Part model, mm, in its own coordinate system. Face numbers are marked on the shaded views. A direction names the side the tool comes from. Coordinates: 2 decimals unless noted, no trailing zeros. Loops run counter-clockwise (first coordinate to the right, second up) from the corner with the lowest first, then second, coordinate; pieces in that order, holes last. Notation, with made-up numbers: (-32, -37.5) -> (-25, -37.5) arc R19 ccw to (-25, -7.5) -> close; hole circle Ø4 at (-35, 29). An arc over 180 degrees is marked (long way). One line per question, with ' | ' between items. Start each with the question number.
1) Drop flat-ended pins along their axis: pin 1 (3 mm diameter, centred on x = 3, z = -2, fed in from -Y); pin 2 (4 mm diameter, centred on x = -2, y = 2.5, fed in from -Z). Give the stop position or say it passes through.
2) 3-axis set-ups, long thin cutter, end or side, ignore diameter. For the marked faces 4 and 5: which of +Z, -Z, +X, -X, +Y, -Y reach the whole face in a straight line?
3) Cut at A-A (z = 4.25). List the corners of the cut face in (x, y).
4) Two-plate mould, pull along Z, no slides. Class the marked faces 1, 2 and 3: released by +Z, released by -Z, zero draft, split by the parting line, or undercut.
5) Probe L1, parallel to X at y = -1.5, z = 1.25; L2, parallel to X at y = 0.5, z = 4; L3, parallel to Z at x = 4.25, y = 0.5. List the from-to ranges inside material, lowest first. Write a range as from..to.
6) Cut at B-B (y = -3). List the corners of the cut face in (x, z), plus the area to 3 significant figures.
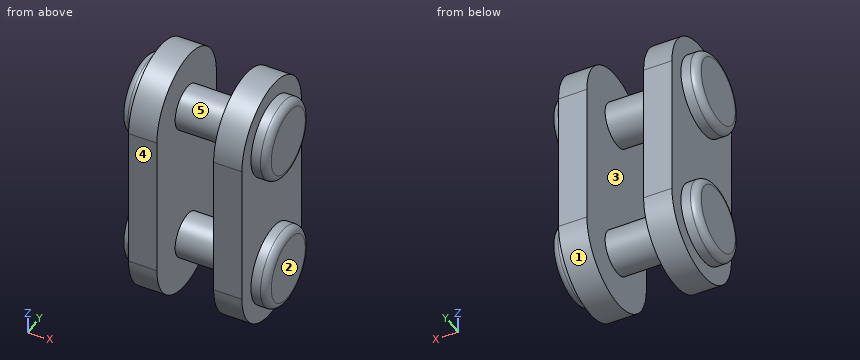
Autodesk Inventor part; units mm, degrees
ref_plane "ZS1_XY" through (0, 0, 0) normal (1, 0, 0) x (0, 0, -1)
ref_plane "ZS1_YZ" through (0, 0, 0) normal (0, 0, -1) x (0, 1, 0)
ref_plane "ZS1_ZX" through (0, 0, 0) normal (0, 1, 0) x (1, 0, 0)
sketch "Skizze_1" plane through (0, 0, 0) normal (0, 1, 0) x (-1, 0, 0)
  line L0 (4, 14.4) -> (2, 14.4)
  line L1 (2, 14.4) -> (2, -4)
  line L2 (2, -4) -> (4, -4)
  line L3 (4, -4) -> (4, 14.4)
extrude "Extrusion1" add sketch "Skizze_1" along normal mid plane 8
sketch "Skizze_2" plane through (0, 0, 0) normal (0, 1, 0) x (-1, 0, 0)
  line L0 (-5.17, 0) -> (0, 0)
  line L1 (5.17, 0) -> (5.17, -2.29)
  arc A0 (4.67, -2.79) -> (5.17, -2.29) centre (4.67, -2.29) ccw
  line L2 (4.67, -2.79) -> (4, -2.79)
  line L3 (4, -2.79) -> (4, -1.55)
  line L4 (4, -1.55) -> (-4, -1.55)
  line L5 (-4, -1.55) -> (-4, -2.79)
  line L6 (-4, -2.79) -> (-4.67, -2.79)
  arc A1 (-5.17, -2.29) -> (-4.67, -2.79) centre (-4.67, -2.29) ccw
  line L7 (-5.17, -2.29) -> (-5.17, 0)
  line L8 (-5.17, 0) -> (5.17, 0)
revolve "Revolution1" add sketch "Skizze_2" angle 360 about axis through (5.17, 0, 0) along (1, 0, 0)
sketch "Skizze_3" plane through (0, 0, 0) normal (0, 1, 0) x (-1, 0, 0)
  line L0 (-5.17, 10.4) -> (0, 10.4)
  line L1 (5.17, 10.4) -> (5.17, 8.11)
  arc A0 (4.67, 7.61) -> (5.17, 8.11) centre (4.67, 8.11) ccw
  line L2 (4.67, 7.61) -> (4, 7.61)
  line L3 (4, 7.61) -> (4, 8.85)
  line L4 (4, 8.85) -> (-4, 8.85)
  line L5 (-4, 8.85) -> (-4, 7.61)
  line L6 (-4, 7.61) -> (-4.67, 7.61)
  arc A1 (-5.17, 8.11) -> (-4.67, 7.61) centre (-4.67, 8.11) ccw
  line L7 (-5.17, 8.11) -> (-5.17, 10.4)
  line L8 (-5.17, 10.4) -> (5.17, 10.4)
revolve "Revolution2" add sketch "Skizze_3" angle 360 about axis through (5.17, 0, 10.4) along (1, 0, 0)
sketch "Skizze_4" plane through (0, 0, 0) normal (0, 1, 0) x (-1, 0, 0)
  line L0 (-2, 14.4) -> (-4, 14.4)
  line L1 (-4, 14.4) -> (-4, -4)
  line L2 (-4, -4) -> (-2, -4)
  line L3 (-2, -4) -> (-2, 14.4)
extrude "Extrusion2" add sketch "Skizze_4" along normal mid plane 8
sketch "Skizze_5" plane through (0, 0, 0) normal (1, 0, 0) x (0, 1, 0)
  line L0 (-20, 30) -> (-20, -40)
  line L1 (-20, -40) -> (10, -40)
  line L2 (10, -40) -> (10, 30)
  line L3 (10, 30) -> (-20, 30)
  arc A0 (4, 10.4) -> (-4, 10.4) centre (0, 10.4) ccw
  line L4 (-4, 10.4) -> (-4, 0)
  arc A1 (-4, 0) -> (4, 0) centre (0, 0) ccw
  line L5 (4, 0) -> (4, 10.4)
extrude "Extrusion3" cut sketch "Skizze_5" along normal mid plane 20
ref_plane "ZS1_XY" through (0, 0, 0) normal (1, 0, 0) x (0, 0, -1)
ref_plane "ZS1_YZ" through (0, 0, 0) normal (0, 0, -1) x (0, 1, 0)
ref_plane "ZS1_ZX" through (0, 0, 0) normal (0, 1, 0) x (1, 0, 0)
ref_plane "ZS2_XY" through (0, 0, 10.4) normal (1, 0, 0) x (0, 0, -1)
ref_plane "ZS2_YZ" through (0, 0, 10.4) normal (0, 0, -1) x (0, 1, 0)
ref_plane "ZS2_ZX" through (0, 0, 10.4) normal (0, 1, 0) x (1, 0, 0)
properties part number "305103-M-KOMP"
Reported:
1) pin 1: stops at y = -3.97 | pin 2: stops at z = -3.97
2) face 4: +Z, -Z, +X, -X, -Y | face 5: none
3) outline: (-4, -4) -> (-2, -4) -> (-2, 4) -> (-4, 4) -> close; (2, -4) -> (4, -4) -> (4, 4) -> (2, 4) -> close
4) face 1: released by -Z | face 2: zero draft | face 3: undercut
5) L1: x = -5.17..-2, 2..5.17 | L2: x = -4..-2, 2..4 | L3: z = -2.74..2.74, 7.66..13.14
6) outline: (-4, -2.65) -> (-2, -2.65) -> (-2, 13.05) -> (-4, 13.05) -> close; (2, -2.65) -> (4, -2.65) -> (4, 13.05) -> (2, 13.05) -> close | area: 62.8 mm²
